```python
from build123d import *

# Parameters (mm, degrees)
SKETCH1_W                      = 278.13
SKETCH1_H                      = 251.191235252
BOSS_EXTRUDE1_DEPTH            = 6.35
DRAFT1_ANGLE                   = -12.5
HOLE1_D                        = 28.575
HOLE1_DEPTH                    = 59.131528827
F_7_0_201_DIAMETER_HOLE1_D     = 5.1054
F_7_0_201_DIAMETER_HOLE1_DEPTH = 59.131528827
BOSS_EXTRUDE2_DEPTH            = 1.27


with BuildPart() as part:
    # Sketch1 → Boss-Extrude1 (new body)
    with BuildSketch(Plane(origin=(191.25417179, 0, 862.691819056), x_dir=(0, 1, 0), z_dir=(0.21643961393810301, 0, 0.9762960071199335))):
        with Locations((145.415, -415.039419658)):
            Rectangle(SKETCH1_W, SKETCH1_H)
    extrude(amount=-BOSS_EXTRUDE1_DEPTH)

    # Draft1
    draft1_faces = [part.faces().sort_by_distance(p)[0] for p in [
        (473.149804226, 145.415, 796.944974464),
    ]]
    draft(draft1_faces, Plane(origin=(191.25417179, 0, 862.691819056), x_dir=(0.9762960071199334, 0, -0.21643961393810301), z_dir=(0.216439613938103, 0, 0.9762960071199333)), DRAFT1_ANGLE)

    # Hole1
    with Locations(Plane(origin=(191.25417179, 0, 862.691819056), x_dir=(0.976296007119934, 0, -0.21643961393809993), z_dir=(0.21643961393809993, 0, 0.9762960071199341))):
        with Locations((348.630068619, 222.25), (508.166081715, 234.95), (508.166081715, 57.15), (348.630068619, 69.85)):
            Hole(HOLE1_D / 2, depth=HOLE1_DEPTH)

    # #7 (0.201) Diameter Hole1
    with Locations(Plane(origin=(191.25417179, 0, 862.691819056), x_dir=(0.9762960071199334, 0, -0.216439613938103), z_dir=(0.21643961393810301, 0, 0.9762960071199335))):
        with Locations((359.982142032, 273.05), (410.782142032, 273.05), (461.582142032, 273.05), (512.382142032, 273.05), (486.982142032, 273.05), (436.182142032, 273.05), (385.382142032, 273.05), (334.582142032, 273.05), (512.382607571, 19.05), (486.982607571, 19.05), (461.582607571, 19.05), (436.182607571, 19.05), (410.782607571, 19.05), (385.382607571, 19.05), (359.982607571, 19.05), (334.582607571, 19.05), (309.182607571, 19.05), (309.182142032, 273.05)):
            Hole(F_7_0_201_DIAMETER_HOLE1_D / 2, depth=F_7_0_201_DIAMETER_HOLE1_DEPTH)

    # Sketch6 → Boss-Extrude2 (add)
    with BuildSketch(Plane(origin=(0, 284.48, 0), x_dir=(1, 0, 0), z_dir=(0, 1, 0))):
        Polygon((473.837, -800.044714287), (473.837, -793.540539371), (717.699608451, -739.477500659), (719.074, -745.676980304), align=None)
    extrude(amount=BOSS_EXTRUDE2_DEPTH)


solid = part.part
```
For this review, take the finished solid that the model builds, in its own axes (mm). Round coordinates to 2 decimals unless told otherwise and drop trailing zeros. Write each loop counter-clockwise with the first axis right and the second up, starting at its lowest first coordinate (ties: lowest second). Pieces come first, ordered by that corner, then holes. Notation, with made-up numbers: (17.25, -14) - (47.25, -14) arc R10 ccw to (47.25, -1) - close; hole circle Ø6 at (32, -7.5). An arc over 180 degrees is marked (long way). Answer as a JSON object with one key per item and string values.
1. For pin 1 Ø3 at (x, y) = (642, 161.5) entering from +Z, flat-tipped, find the tip position at first contact; note if it passes through.
Response values:
{"pin 1": "stops at z = 763.1"}
2. We need section D-D on y = 37. Give the boundary of the cut face in (x, z), then the cut area to 3 significant figures.
Response values:
{"outline": "(473.84, 793.54) - (717.7, 739.48) - (719.07, 745.68) - (473.84, 800.04) - close", "area": "1,590 mm2"}
3. Draft analysis for pull direction X (two halves, no side actions). For faces 1 (the face through (567.13, 275.58, 776.06)), 2 (the face through (564.503, 18.072, 776.647)), 3 (the face through (597, 6.35, 769)), 4 (the face through (594.061, 144.094, 766.887)), state which applies: +X half, -X half, draft (parallel to the pull), parting line (faces both ways), or undercut.
Response values:
{"face 1": "undercut", "face 2": "undercut", "face 3": "draft", "face 4": "-X half"}
4. We need section B-B on x = 524.5. Count the separate pieces of the cut face and the enclosed holes in it, then the cut area to 3 significant figures.
Response values:
{"separate pieces": "3", "enclosed holes": "0", "area": "1,490 mm2"}
5. We need section C-C on y = 243.5. Give the boundary of the cut face in (x, z).
Response values:
{"outline": "(473.84, 793.54) - (674.82, 748.98) - (676.2, 755.18) - (473.84, 800.04) - close; (697.18, 744.03) - (717.7, 739.48) - (719.07, 745.68) - (698.55, 750.23) - close"}
6. To check wall thickness, follow line 1 along Y through (x, z) = (684.5, 749); line 2 along Y through (x, z) = (682.5, 749); line 3 along Z through (x, y) = (675, 126). State the ranges of each line that lie inside material, in increasing order.
Response values:
{"line 1": "y = 6.35 to 43, 71.3 to 220.8, 249.1 to 285.75", "line 2": "y = 6.35 to 43.42, 70.88 to 221.22, 248.68 to 285.75", "line 3": "z = 748.94 to 755.45"}
7. We need section A-A on y = 75.5. Give the boundary of the cut face in (x, z), then the cut area to 3 significant figures.
Response values:
{"outline": "(473.84, 793.54) - (517.43, 783.88) - (518.81, 790.07) - (473.84, 800.04) - close; (543.06, 778.19) - (717.7, 739.48) - (719.07, 745.68) - (544.43, 784.39) - close", "area": "1,420 mm2"}
